The figure shows three views and two pictorial views of one solid part (mm, origin at its lowest corner). Answer the questions. A direction names the side the tool comes from. Give positions to 0.01 mm unless a question says otherwise; leave off trailing zeros. Order: outer loops, then holes, each group sorted by start corner. A loop starts at its lowest first (then second) coordinate and runs counter-clockwise, first axis right, second up. Notation, with made-up numbers: (77.25, 72) - (90.25, 72) arc R25 cw to (90.25, 98) - close; hole circle Ø5 at (47.25, -25). An arc over 180 degrees is marked (long way). Answer as a JSON object with one key per item and string values. Group by question number.
Q1. A cutting plane is placed at B-B, the plane y = 3.5. Count the separate pieces of the cut face and the enclosed holes in it.
Q2. For the marked faces 1 and 2, determine the directions among +Z, -Z, +X, -X, +Y, -Y from which every point of the face is accessible in a straight line to the end or side of a thin tool.
Q3. The mould has two halves that part along Y. Classify the marked faces 3, 4 and 5: released by +Y, released by -Y, zero draft, split by the parting line, or undercut.
Q4. Given pin 1 (1.5 mm diameter, centred on y = 2, z = 3.5, fed in from -X); pin 2 (3 mm diameter, centred on x = 20.5, z = 3, fed in from +Y), each flat-ended and moving along its own axis, determine where each tip first touches the part or whether it passes through.
Q5. Consider line 1 (Z direction, x = 16, y = 5.5); line 2 (X direction, y = 12, z = 0.75); line 3 (X direction, y = 4, z = 4.75). Determine where each line is inside the solid, lowest interval first.
Q6. A cutting plane is placed at A-A, the plane y = 13.5. Give the vertices of the cut face in (x, z).
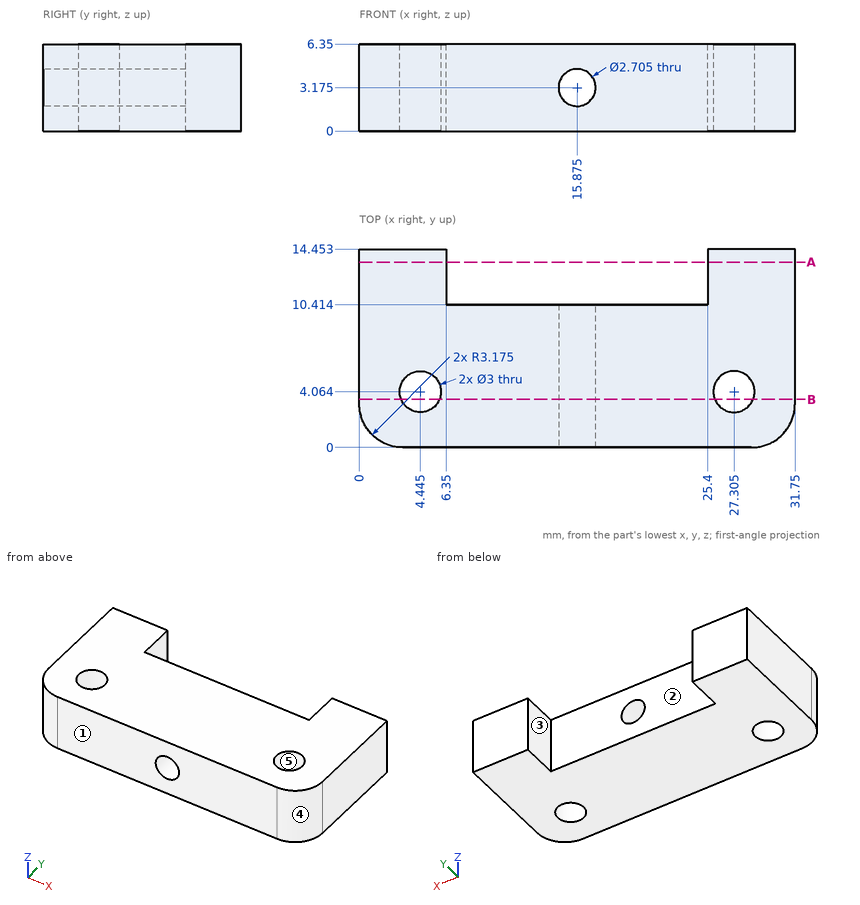
Reply:
{
 "1": {"separate pieces": "3", "enclosed holes": "1"},
 "2": {"face 1": "+Z, -Z, +X, -X, -Y", "face 2": "+Z, -Z, +Y"},
 "3": {"face 3": "zero draft", "face 4": "released by -Y", "face 5": "undercut"},
 "4": {"pin 1": "stops at x = 0.03", "pin 2": "stops at y = 10.41"},
 "5": {"line 1": "z = 0 to 1.83, 4.52 to 6.35", "line 2": "x = 0 to 6.35, 25.4 to 31.75", "line 3": "x = 0 to 2.95, 5.94 to 25.81, 28.8 to 31.75"},
 "6": {"outline": "(0, 0) - (6.35, 0) - (6.35, 6.35) - (0, 6.35) - close; (25.4, 0) - (31.75, 0) - (31.75, 6.35) - (25.4, 6.35) - close"}
}
